from build123d import *

# Parameters (mm, degrees)
SKETCH1_W           = 80
SKETCH1_H           = 80
BOSS_EXTRUDE1_DEPTH = 80
SKETCH2_W           = 75
SKETCH2_H           = 75
CUT_EXTRUDE1_DEPTH  = 75
SKETCH3_R           = 2.5
CUT_EXTRUDE2_DEPTH  = 50
SKETCH4_R           = 2.5
CUT_EXTRUDE3_DEPTH  = 50
SKETCH5_R           = 22.5
CUT_EXTRUDE4_DEPTH  = 50
SKETCH8_W           = 80
SKETCH8_H           = 80
BOSS_EXTRUDE2_DEPTH = 5
SKETCH9_R           = 2.5
CUT_EXTRUDE5_DEPTH  = 5
SKETCH10_W          = 5
SKETCH10_H          = 10
CUT_EXTRUDE6_DEPTH  = 75
SKETCH11_W          = 5
SKETCH11_H          = 75
CUT_EXTRUDE7_DEPTH  = 75


with BuildPart() as part:
    # Sketch1 → Boss-Extrude1 (new body)
    with BuildSketch(Plane.XY):
        Rectangle(SKETCH1_W, SKETCH1_H)
    extrude(amount=BOSS_EXTRUDE1_DEPTH)

    # Sketch2 → Cut-Extrude1 (cut)
    with BuildSketch(Plane.XY.offset(80)):
        with Locations((-2.5, -2.5)):
            Rectangle(SKETCH2_W, SKETCH2_H)
    extrude(amount=-CUT_EXTRUDE1_DEPTH, mode=Mode.SUBTRACT)

    # Sketch3 → Cut-Extrude2 (cut)
    with BuildSketch(Plane.ZY.offset(-35)):
        with Locations((55, -17.5)):
            Circle(SKETCH3_R)
        with Locations((20, -17.5)):
            Circle(SKETCH3_R)
        with Locations((20, 17.5)):
            Circle(SKETCH3_R)
        with Locations((55, 17.5)):
            Circle(SKETCH3_R)
    extrude(amount=-CUT_EXTRUDE2_DEPTH, mode=Mode.SUBTRACT)

    # Sketch4 → Cut-Extrude3 (cut)
    with BuildSketch(Plane.XZ.offset(-35)):
        with Locations((-26, 66)):
            Circle(SKETCH4_R)
        with Locations((21, 66)):
            Circle(SKETCH4_R)
        with Locations((-26, 19)):
            Circle(SKETCH4_R)
        with Locations((21, 19)):
            Circle(SKETCH4_R)
    extrude(amount=-CUT_EXTRUDE3_DEPTH, mode=Mode.SUBTRACT)

    # Sketch5 → Cut-Extrude4 (cut)
    with BuildSketch(Plane.XZ.offset(-35)):
        with Locations((-2.5, 42.5)):
            Circle(SKETCH5_R)
    extrude(amount=-CUT_EXTRUDE4_DEPTH, mode=Mode.SUBTRACT)

    # Sketch8 → Boss-Extrude2 (add)
    with BuildSketch(Plane.ZY.offset(40)):
        with Locations((40, 0)):
            Rectangle(SKETCH8_W, SKETCH8_H)
    extrude(amount=BOSS_EXTRUDE2_DEPTH)

    # Sketch9 → Cut-Extrude5 (cut)
    with BuildSketch(Plane.ZY.offset(45)):
        with Locations((22.5, 17.5)):
            Circle(SKETCH9_R)
        with Locations((57.5, 17.5)):
            Circle(SKETCH9_R)
        with Locations((22.5, -17.5)):
            Circle(SKETCH9_R)
        with Locations((57.5, -17.5)):
            Circle(SKETCH9_R)
    extrude(amount=-CUT_EXTRUDE5_DEPTH, mode=Mode.SUBTRACT)

    # Sketch10 → Cut-Extrude6 (cut)
    with BuildSketch(Plane.XZ.offset(40)):
        with Locations((-42.5, 75)):
            Rectangle(SKETCH10_W, SKETCH10_H)
        with Locations((-42.5, 5)):
            Rectangle(SKETCH10_W, SKETCH10_H)
    extrude(amount=-CUT_EXTRUDE6_DEPTH, mode=Mode.SUBTRACT)

    # Sketch11 → Cut-Extrude7 (cut)
    with BuildSketch(Plane.ZY.offset(40)):
        with Locations((2.5, -2.5)):
            Rectangle(SKETCH11_W, SKETCH11_H)
    extrude(amount=-CUT_EXTRUDE7_DEPTH, mode=Mode.SUBTRACT)


solid = part.part
Check sheet for the modelled part. Datum: model origin and axes. Units: mm. A direction names the side the tool comes from. Round coordinates to 2 decimals unless told otherwise and drop trailing zeros. Order: outer loops, then holes, each group sorted by start corner. A loop starts at its lowest first (then second) coordinate and runs counter-clockwise, first axis right, second up. Notation, with made-up numbers: M 9.25,83 L 24.25,83 A24 ccw 24.25,110 Z; hole C 42,31.5 d2. An arc over 180 degrees is marked long. One line per item, written item: value. Start each with the question number.
1. Section check B-B on y = -17.5. Enter the section's corners in (x, z), and give its area (3 significant figures).
2. Section check A-A on z = 42.5. Enter the section's corners in (x, y), and give its area (3 significant figures).
3. Scan lines: line 1 along Y through (x, z) = (-41.15, 22.5); line 2 along Z through (x, y) = (-2, 39); line 3 along X through (y, z) = (-18, 40). Record each from-to range of solid material in increasing order.
4. Gauge pin test, flat ends, axial feed: P1, Ø1, axis at x = 15.5, z = 54, coming from the -Y side; P2, Ø2.5, axis at x = -41.5, y = 14.5, coming from the +Z side; P3, Ø6, axis at y = 17.5, z = 57.5, coming from the -X side; P4, Ø3, axis at x = 9.5, z = 71.5, coming from the -Y side. Record the tip position at first contact, or that the pin passes through.
5. Access from +Z, -Z, +X, -X, +Y, -Y to the whole of each face (thin tool, end or side, straight path). Record for faces 3 (the flat face through (-43, -3, 10)), 4 (the cylindrical face through (37.47, -18.46, 57.31)), 5 (the cylindrical face through (-42.54, 19.19, 20.66)), 6 (the flat face through (35, -2, 39)).
6. Section check C-C on x = 3. Enter the section's corners in (y, z), and give its area (3 significant figures).
7. Release check for a two-part mould opening along X. For faces 1 (the cylindrical face through (-28.5, 37.5, 66.1)), 2 (the cylindrical face through (37.5, -17.4, 17.5)) record: released by +X, released by -X, zero draft, split by the parting line, or undercut.
8. Section check D-D on y = 23. Enter the section's corners in (x, z).
Results found:
1. outline: M -45,10 L -40,10 L -40,20 L -45,20 Z; M -45,25 L -40,25 L -40,55 L -45,55 Z; M -45,60 L -40,60 L -40,70 L -45,70 Z; M 35,0 L 40,0 L 40,17.5 L 35,17.5 Z; M 35,22.5 L 40,22.5 L 40,52.5 L 35,52.5 Z; M 35,57.5 L 40,57.5 L 40,80 L 35,80 Z
1. area: 600 mm^2
2. outline: M -45,-40 L -40,-40 L -40,35 L -25,35 L -25,40 L -45,40 Z; M 20,35 L 35,35 L 35,-40 L 40,-40 L 40,40 L 20,40 Z
2. area: 950 mm^2
3. line 1: -40 to -20, -15 to 15, 20 to 40
3. line 2: 0 to 20.01, 64.99 to 80
3. line 3: -45 to -40, 35 to 40
4. P1: through
4. P2: z = 70
4. P3: x = -45
4. P4: y = 35
5. face 3: -Z, -X, -Y
5. face 4: +X
5. face 5: -X
5. face 6: +Z, -Z, -Y
6. outline: M 35,0 L 40,0 L 40,20.68 L 35,20.68 Z; M 35,64.32 L 40,64.32 L 40,80 L 35,80 Z
6. area: 182 mm^2
7. face 1: undercut
7. face 2: zero draft
8. outline: M -45,10 L -40,10 L -40,70 L -45,70 Z; M 35,0 L 40,0 L 40,80 L 35,80 Z
